Geometry check sheet. Reference: the model listing, model coordinates, mm. Round coordinates to 2 decimals unless told otherwise and drop trailing zeros. Order: outer loops, then holes, each group sorted by start corner. A loop starts at its lowest first (then second) coordinate and runs counter-clockwise, first axis right, second up. Notation, with made-up numbers: (25.5, 24) - (58.5, 24) arc R31 cw to (58.5, 53) - close; hole circle Ø11 at (-6, -23). An arc over 180 degrees is marked (long way). Use a Markdown table: item, result. Add a question column.
(1) Mould release check, pull along Z, two halves, no side actions. Record for faces 1 (the face through (-3, 4, 3)), 2 (the face through (5.47, 1.97, 9.31)), 3 (the face through (6.163, 1.972, -8.484)), 4 (the face through (0.66, 1.972, -14.985)): released by +Z, released by -Z, zero draft, split by the parting line, or undercut.
(2) Section check A-A on z = 0. Record the boundary of the cut face in (x, y), then the cut area to 3 significant figures.
(3) Section check D-D on z = 9. Record the boundary of the cut face in (x, y).
(4) Gauge pin test, flat end, axial feed: P1, Ø2, axis at x = -6.5, y = 2, coming from the +Z side. Record the tip position at first contact, or that the pin passes through.
(5) Section check C-C on y = 0.75. Record the boundary of the cut face in (x, z).
(6) Section check B-B on x = 1.75. Record the boundary of the cut face in (y, z).
(7) Thickness scan on line 1 along Z through (x, y) = (4.5, 1.5); line 2 along X through (y, z) = (2.1, -2.25); line 3 along X through (y, z) = (0.9, -7). Record the ranges inside material, lowest first. Write a range as [from, to].
```python
from build123d import *

# Parameters (mm, degrees)
CROQUIS1_R                       = 15
CROQUIS1_R_2                     = 4
SALIENTE_EXTRUIR1_DEPTH          = 4
TALADRO_DE_MARGEN_PARA_M31_D     = 3.6
TALADRO_DE_MARGEN_PARA_M31_DEPTH = 5
TALADRO_DE_MARGEN_PARA_M31_TIP   = 1.081549114


with BuildPart() as part:
    # Croquis1 → Saliente-Extruir1 (new body)
    with BuildSketch(Plane(origin=(0, 0, 0), x_dir=(-1, 0, 0), z_dir=(0, 1, 0))):
        with Locations(Location((0, 0, 0), (0, 0, 90))):
            Circle(CROQUIS1_R)
        with Locations(Location((0, 0, 0), (0, 0, 90))):
            Circle(CROQUIS1_R_2, mode=Mode.SUBTRACT)
    extrude(amount=SALIENTE_EXTRUIR1_DEPTH)

    # Taladro de margen para M31
    with Locations(Plane(origin=(0, 4, 0), x_dir=(-1, 0, 0), z_dir=(0, 1, 0))):
        with Locations((-4.5, 7.794228634), (9, 0), (-4.5, -7.794228634), (0, 0)):
            Hole(TALADRO_DE_MARGEN_PARA_M31_D / 2, depth=TALADRO_DE_MARGEN_PARA_M31_DEPTH)
            with Locations((0, 0, -(TALADRO_DE_MARGEN_PARA_M31_DEPTH + TALADRO_DE_MARGEN_PARA_M31_TIP / 2))):  # 118° drill point
                Cone(0, TALADRO_DE_MARGEN_PARA_M31_D / 2, TALADRO_DE_MARGEN_PARA_M31_TIP, mode=Mode.SUBTRACT)


solid = part.part
```
Check sheet entries:
| question | item | result |
|---|---|---|
| 1 | face 1 | zero draft |
| 1 | face 2 | undercut |
| 1 | face 3 | undercut |
| 1 | face 4 | split by the parting line |
| 2 | outline | (-15, 0) - (-10.8, 0) - (-10.8, 4) - (-15, 4) - close; (-7.2, 0) - (-4, 0) - (-4, 4) - (-7.2, 4) - close; (4, 0) - (15, 0) - (15, 4) - (4, 4) - close |
| 2 | area | 73.6 mm2 |
| 3 | outline | (-12, 0) - (3.16, 0) - (3.16, 4) - (-12, 4) - close; (5.84, 0) - (12, 0) - (12, 4) - (5.84, 4) - close |
| 4 | P1 | stops at z = 13.96 |
| 5 | outline | circle Ø30 at (0, 0); hole circle Ø3.6 at (-9, 0); hole circle Ø8 at (0, 0); hole circle Ø3.6 at (4.5, -7.79); hole circle Ø3.6 at (4.5, 7.79) |
| 6 | outline | (0, -14.9) - (4, -14.9) - (4, -3.6) - (0, -3.6) - close; (0, 3.6) - (4, 3.6) - (4, 14.9) - (0, 14.9) - close |
| 7 | line 1 | z = [-14.31, -9.59], [-5.99, 5.99], [9.59, 14.31] |
| 7 | line 2 | x = [-14.83, -3.31], [3.31, 14.83] |
| 7 | line 3 | x = [-13.27, 2.88], [6.12, 13.27] |
